Design review of the part built by this model. Coordinates are the model's own, in mm. Face numbers are marked on the shaded views. A direction names the side the tool comes from. Coordinates: 2 decimals unless noted, no trailing zeros. Loops run counter-clockwise (first coordinate to the right, second up) from the corner with the lowest first, then second, coordinate; pieces in that order, holes last. Notation, with made-up numbers: (-28, 44.25) - (24, 44.25) arc R29 cw to (24, 83.25) - close; hole circle Ø1 at (76.25, 37.25). An arc over 180 degrees is marked (long way). One line per question, with ' | ' between items.
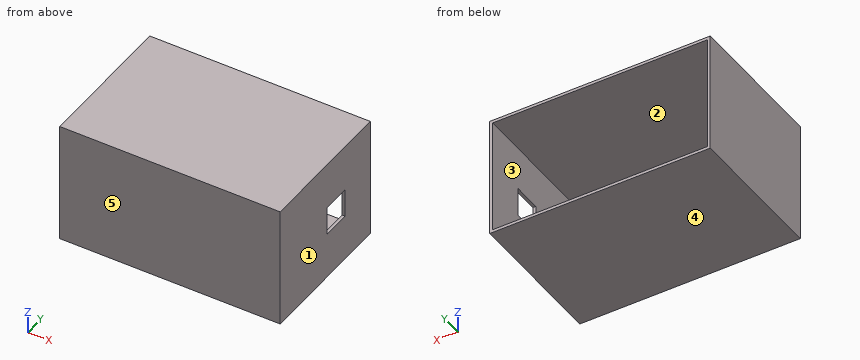
Autodesk Inventor part; units mm, degrees
ref_plane "YZ Plane" through (0, 0, 0) normal (1, 0, 0) x (0, 1, 0)
ref_plane "XZ Plane" through (0, 0, 0) normal (0, 1, 0) x (-1, 0, 0)
ref_plane "XY Plane" through (0, 0, 0) normal (0, 0, 1) x (1, 0, 0)
sketch "Sketch1" plane through (0, 0, 0) normal (0, 1, 0) x (-1, 0, 0)
  line L0 (-38, 21) -> (38, 21)
  line L1 (38, 21) -> (38, -21)
  line L2 (38, -21) -> (-38, -21)
  line L3 (-38, -21) -> (-38, 21)
  line L4 (-38, 21) -> (38, -21) construction
  line L5 (38, 21) -> (-38, -21) construction
  point P0 (0, 0)
  dimension "d0" = 42
  dimension "d1" = 76
extrude "Extrusion1" add sketch "Sketch1" along normal blind 50
sketch "Sketch2" plane through (0, 50, 0) normal (0, 1, 0) x (1, 0, 0)
  point P0 (0, 0)
sketch "Sketch3" plane through (0, 50, 0) normal (0, 1, 0) x (1, 0, 0)
  line L0 (-37, -20) -> (37, -20)
  line L1 (37, -20) -> (37, 20)
  line L2 (37, 20) -> (-37, 20)
  line L3 (-37, 20) -> (-37, -20)
  line L4 (-37, -20) -> (37, 20) construction
  line L5 (37, -20) -> (-37, 20) construction
  point P0 (0, 0)
  dimension "d4" = 40
  dimension "d5" = 74
extrude "Extrusion2" cut sketch "Sketch3" against normal blind 48
sketch "Sketch4" plane through (38, 0, 21) normal (1, 0, 0) x (0, 0, -1)
  line L0 (26, 74) -> (16, 74)
  line L1 (16, 74) -> (16, 26)
  line L2 (16, 26) -> (26, 26)
  line L3 (26, 26) -> (26, 74)
  line L4 (0, 50) -> (42, 50)
  line L5 (26, 74) -> (16, 26) construction
  line L6 (16, 74) -> (26, 26) construction
  line L7 (16, 26) -> (26, 26)
  line L8 (26, 26) -> (26, 35.9645)
  line L9 (26, 35.9645) -> (16, 35.9645)
  line L10 (16, 35.9645) -> (16, 26)
  point P0 (21, 0)
  point P1 (21, 50)
  dimension "d8" = 10
  dimension "d9" = 48
  dimension "d10" = 10
extrude "Extrusion3" cut sketch "Sketch4" against normal blind 20 contours L3 L2 L1 L9
properties part number "mcu_place"
Q1. Take a section at A-A (z = -3.5). Give the boundary of the cut face in (x, y).
Returned:
outline: (-38, 0) - (38, 0) - (38, 26) - (37, 26) - (37, 2) - (-37, 2) - (-37, 50) - (-38, 50) - close; (37, 35.96) - (38, 35.96) - (38, 50) - (37, 50) - close
Q2. Take a section at C-C (y = 40.5). Give the boundary of the cut face in (x, z).
Returned:
outline: (-38, -21) - (38, -21) - (38, 21) - (-38, 21) - close; hole (-37, -20) - (37, -20) - (37, 20) - (-37, 20) - close
Q3. Take a section at B-B (x = 32). Give the boundary of the cut face in (y, z).
Returned:
outline: (0, -21) - (50, -21) - (50, -20) - (2, -20) - (2, 20) - (50, 20) - (50, 21) - (0, 21) - close
Q4. To check wall thickness, follow line 1 along Z through (x, y) = (-9.5, 20.5); line 2 along X through (y, z) = (3.5, 2.5); line 3 along Y through (x, z) = (-19, -17). State the ranges of each line that lie inside material, in increasing order.
Returned:
line 1: z = -21 to -20, 20 to 21 | line 2: x = -38 to -37, 37 to 38 | line 3: y = 0 to 2
Q5. Draft analysis for pull direction Z (two halves, no side actions). For the marked faces 3, 4 and 5, state which applies: +Z half, -Z half, draft (parallel to the pull), parting line (faces both ways), or undercut.
Returned:
face 3: undercut | face 4: -Z half | face 5: draft
Q6. Take a section at D-D (y = 34). Give the boundary of the cut face in (x, z).
Returned:
outline: (-38, -21) - (38, -21) - (38, -5) - (37, -5) - (37, -20) - (-37, -20) - (-37, 20) - (37, 20) - (37, 5) - (38, 5) - (38, 21) - (-38, 21) - close
Q7. For pin 1 (8 mm diameter, centred on x = -11.5, z = 6, fed in from +Y), flat-tipped, find the tip position at first contact; note if it passes through.
Returned:
pin 1: stops at y = 2
Q8. Tool access review of the marked faces 1 and 2: name each direction out of +Z, -Z, +X, -X, +Y, -Y from which nothing blocks a thin tool from reaching the whole face with its end or side.
Returned:
face 1: +Z, -Z, +X, +Y, -Y | face 2: +Y
